from build123d import *

# Parameters (mm, degrees)
SKETCH1_R           = 1.6
BOSS_EXTRUDE1_DEPTH = 3
SKETCH2_W           = 10
SKETCH2_H           = 10
BOSS_EXTRUDE2_DEPTH = 42
CHAMFER1_SIZE       = 5
SKETCH3_R           = 2.1
CUT_EXTRUDE1_DEPTH  = 52
SKETCH4_R           = 2.65
CUT_EXTRUDE2_DEPTH  = 0.5
SKETCH5_W           = 3
SKETCH5_H           = 43
BOSS_EXTRUDE3_DEPTH = 75
SKETCH6_W           = 3
SKETCH6_H           = 3.9
BOSS_EXTRUDE4_DEPTH = 2
SKETCH7_W           = 3
SKETCH7_H           = 68.8
BOSS_EXTRUDE5_DEPTH = 5
SKETCH8_R           = 1.5
CUT_EXTRUDE3_DEPTH  = 5
SKETCH9_W           = 3
SKETCH9_H           = 68.8
BOSS_EXTRUDE6_DEPTH = 15
SKETCH10_R          = 6
CUT_EXTRUDE4_DEPTH  = 10
SKETCH11_W          = 3
SKETCH11_H          = 68.8
BOSS_EXTRUDE7_DEPTH = 45


with BuildPart() as part:
    # Sketch1 → Boss-Extrude1 (new body)
    with BuildSketch(Plane(origin=(0, 0, 0), x_dir=(1, 0, 0), z_dir=(0, 1, 0))):
        Polygon((-6.512396694, 9.685950413), (1.487603306, 9.685950413), (26.487603306, 9.685950413), (26.487603306, -40.314049587), (1.487603306, -40.314049587), (-6.512396694, -40.314049587), align=None)
        with Locations(Location((-1.962396694, -35.764049587, 0), (0, 0, 270))):
            Circle(SKETCH1_R, mode=Mode.SUBTRACT)
        with Locations(Location((-1.962396694, 5.135950413, 0), (0, 0, 270))):
            Circle(SKETCH1_R, mode=Mode.SUBTRACT)
    extrude(amount=BOSS_EXTRUDE1_DEPTH)

    # Sketch2 → Boss-Extrude2 (add)
    with BuildSketch(Plane(origin=(0, 3, 0), x_dir=(1, 0, 0), z_dir=(0, 1, 0))):
        with Locations((21.487603306, -35.314049587)):
            Rectangle(SKETCH2_W, SKETCH2_H)
        with Locations((21.487603306, 4.685950413)):
            Rectangle(SKETCH2_W, SKETCH2_H)
    extrude(amount=BOSS_EXTRUDE2_DEPTH)

    # Chamfer1
    chamfer1_edges = [part.edges().sort_by_distance(p)[0] for p in [
        (21.487603306, 3, 30.314049587),
        (16.487603306, 3, 35.314049587),
        (16.487603306, 3, -4.685950413),
        (21.487603306, 3, 0.314049587),
    ]]
    chamfer(chamfer1_edges, length=CHAMFER1_SIZE)

    # Sketch3 → Cut-Extrude1 (cut)
    with BuildSketch(Plane(origin=(0, 45, 0), x_dir=(1, 0, 0), z_dir=(0, 1, 0))):
        with Locations(Location((22.537603306, -36.364049587, 0), (0, 0, 270))):
            Circle(SKETCH3_R)
        with Locations(Location((22.537603306, 5.735950413, 0), (0, 0, 270))):
            Circle(SKETCH3_R)
    extrude(amount=-CUT_EXTRUDE1_DEPTH, mode=Mode.SUBTRACT)

    # Sketch4 → Cut-Extrude2 (cut)
    with BuildSketch(Plane(origin=(0, 45, 0), x_dir=(1, 0, 0), z_dir=(0, 1, 0))):
        with Locations(Location((22.537603306, -36.364049587, 0), (0, 0, 270))):
            Circle(SKETCH4_R)
        with Locations(Location((22.537603306, 5.735950413, 0), (0, 0, 270))):
            Circle(SKETCH4_R)
    cut_extrude2 = extrude(amount=-CUT_EXTRUDE2_DEPTH, mode=Mode.SUBTRACT)

    # Mirror1: Cut-Extrude2 across plane
    add(cut_extrude2.mirror(Plane(origin=(0, 22.5, 0), x_dir=(0, 0, 1), z_dir=(0, -1, 0))), mode=Mode.SUBTRACT)

    # Sketch5 → Boss-Extrude3 (add)
    with BuildSketch(Plane.XY.offset(40.314049587)):
        with Locations((24.987603306, 21.5)):
            Rectangle(SKETCH5_W, SKETCH5_H)
    extrude(amount=BOSS_EXTRUDE3_DEPTH)

    # Sketch6 → Boss-Extrude4 (add)
    with BuildSketch(Plane(origin=(0, 43, 0), x_dir=(1, 0, 0), z_dir=(0, 1, 0))):
        with Locations((24.987603306, -44.564049587)):
            Rectangle(SKETCH6_W, SKETCH6_H)
    extrude(amount=BOSS_EXTRUDE4_DEPTH)

    # Sketch7 → Boss-Extrude5 (add)
    with BuildSketch(Plane(origin=(0, 43, 0), x_dir=(1, 0, 0), z_dir=(0, 1, 0))):
        with Locations((24.987603306, -80.914049587)):
            Rectangle(SKETCH7_W, SKETCH7_H)
    extrude(amount=BOSS_EXTRUDE5_DEPTH)

    # Sketch8 → Cut-Extrude3 (cut)
    with BuildSketch(Plane.ZY.offset(-23.487603306)):
        with Locations(Location((52.714049587, 34.5, 0), (0, 0, 270))):
            Circle(SKETCH8_R)
    extrude(amount=-CUT_EXTRUDE3_DEPTH, mode=Mode.SUBTRACT)

    # Sketch9 → Boss-Extrude6 (add)
    with BuildSketch(Plane(origin=(0, 48, 0), x_dir=(1, 0, 0), z_dir=(0, 1, 0))):
        with Locations((24.987603306, -80.914049587)):
            Rectangle(SKETCH9_W, SKETCH9_H)
    extrude(amount=BOSS_EXTRUDE6_DEPTH)

    # Sketch10 → Cut-Extrude4 (cut)
    with BuildSketch(Plane.ZY.offset(-23.487603306)):
        with Locations(Location((97.714049587, 43, 0), (0, 0, 270))):
            Circle(SKETCH10_R)
    extrude(amount=-CUT_EXTRUDE4_DEPTH, mode=Mode.SUBTRACT)

    # Sketch11 → Boss-Extrude7 (add)
    with BuildSketch(Plane(origin=(0, 63, 0), x_dir=(1, 0, 0), z_dir=(0, 1, 0))):
        with Locations((24.987603306, -80.914049587)):
            Rectangle(SKETCH11_W, SKETCH11_H)
    extrude(amount=BOSS_EXTRUDE7_DEPTH)


solid = part.part
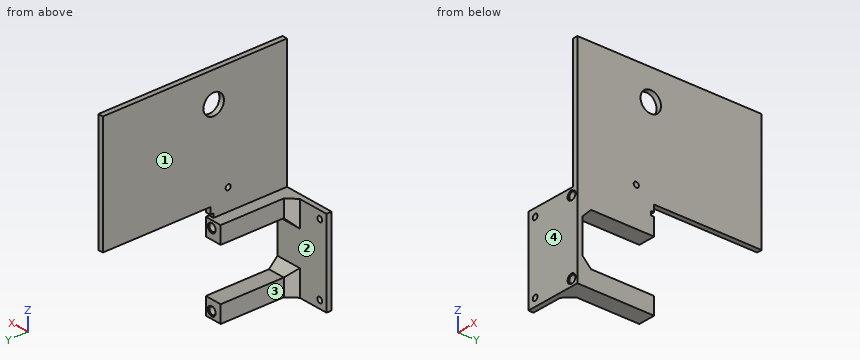
Design review of the part built by this model. Coordinates are the model's own, in mm. Face numbers are marked on the shaded views. A direction names the side the tool comes from. Give positions to 0.01 mm unless a question says otherwise; leave off trailing zeros. Write each loop counter-clockwise with the first axis right and the second up, starting at its lowest first coordinate (ties: lowest second). Pieces come first, ordered by that corner, then holes. Notation, with made-up numbers: M 33,8.25 L 89,8.25 A23 ccw 89,26.25 Z; hole C 23.25,57 d6. An arc over 180 degrees is marked long. Answer as a JSON object with one key per item and string values. Group by question number.
1) We need section D-D (z = 73.5). Give the boundary of the cut face in (x, y).
2) Clearance check with flat-ended pins moving along their axes: pin 1 Ø1.6 at (x, z) = (23.5, -7) entering from +Y; pin 2 Ø0.7 at (x, z) = (25, 41.5) entering from +Y; pin 3 Ø1 at (x, z) = (21, 30.5) entering from +Y; pin 4 Ø3.5 at (x, z) = (22.54, 36.36) entering from -Y. State where each tip first meets the part, or that it passes through.
3) We need section B-B (y = 17). Give the boundary of the cut face in (x, z).
4) We need section A-A (y = 34.5). Give the boundary of the cut face in (x, z), and give its area (3 significant figures).
5) Tool access review of the marked faces 1, 2, 3 and 4: name each direction out of +Z, -Z, +X, -X, +Y, -Y from which nothing blocks a thin tool from reaching the whole face with its end or side.
6) We need section C-C (x = 1.5). Give the boundary of the cut face in (y, z), and give its area (3 significant figures).
7) For line 1 along X through (y, z) = (5.5, 92.5); line 2 along Y through (x, z) = (4, 22); line 3 along Y through (x, z) = (18.5, 34), list the stretches that pass through material, from the lowest coordinate up.
Answer key:
{
 "1": {"outline": "M 23.49,0 L 26.49,0 L 26.49,108 L 23.49,108 Z"},
 "2": {"pin 1": "stops at y = 44.5", "pin 2": "stops at y = 43", "pin 3": "stops at y = 45", "pin 4": "passes through"},
 "3": {"outline": "M 16.49,-9.69 L 26.49,-9.69 L 26.49,0.31 L 16.49,0.31 Z; M 16.49,30.31 L 26.49,30.31 L 26.49,115.31 L 23.49,115.31 L 23.49,40.31 L 16.49,40.31 Z; hole C 22.54,-5.74 d4.2; hole C 22.54,36.36 d4.2"},
 "4": {"outline": "M 16.49,-9.69 L 26.49,-9.69 L 26.49,0.31 L 16.49,0.31 Z; M 16.49,30.31 L 26.49,30.31 L 26.49,51.21 L 23.49,51.21 L 23.49,40.31 L 16.49,40.31 Z; M 23.49,54.21 L 26.49,54.21 L 26.49,115.31 L 23.49,115.31 Z; hole C 22.54,-5.74 d4.2; hole C 22.54,36.36 d4.2", "area": "388 mm²"},
 "5": {"face 1": "+Z, -X, +Y, -Y", "face 2": "-X, +Y", "face 3": "+Z, -Z, -X, +Y", "face 4": "+Z, -Z, +X, -X, -Y"},
 "6": {"outline": "M 0,-9.69 L 3,-9.69 L 3,40.31 L 0,40.31 Z", "area": "150 mm²"},
 "7": {"line 1": "x = 23.49 to 26.49", "line 2": "y = 0 to 3", "line 3": "y = 0 to 45"}
}
